Autodesk Fusion 360 part; units mm, degrees
sketch "Sketch1" plane through (0, 0, 0) normal (0, 0, 1) x (1, 0, 0)
  line L0 (40, -70) -> (-40, -70)
  line L1 (-40, -70) -> (-40, 70)
  line L2 (-40, 70) -> (40, 70)
  line L3 (40, 70) -> (40, -70)
  line L4 (40, -70) -> (-40, 70) construction
  line L5 (-40, -70) -> (40, 70) construction
extrude "Extrude1" add sketch "Sketch1" along normal blind 60
sketch "Sketch2" plane through (40, 0, 0) normal (1, 0, 0) x (0, 1, 0)
  line L0 (-70, 0) -> (70, 0)
  line L1 (70, 0) -> (70, 60)
  line L2 (70, 60) -> (-70, 60)
  line L3 (-70, 60) -> (-70, 0)
fillet "Fillet1" radius 10 3 edges at (40, 0, 60) (40, -70, 30) (40, 70, 30)
extrude "Extrude2" add sketch "Sketch2" along normal blind 10
extrude "Extrude3" add 1 faces at (-16.6667, 70, 20) along direction (0, 1, 0) blind 20
sketch "Sketch3" plane through (0, 0, 0) normal (1, 0, 0) x (0, 1, 0)
  line L0 (-1.1501, 56.847) -> (-18.8499, 56.847)
  line L1 (-18.8499, 56.847) -> (-18.8499, 63.153)
  line L2 (-18.8499, 63.153) -> (-1.1501, 63.153)
  line L3 (-1.1501, 63.153) -> (-1.1501, 56.847)
  line L4 (-1.1501, 56.847) -> (-18.8499, 63.153) construction
  line L5 (-18.8499, 56.847) -> (-1.1501, 63.153) construction
  point P0 (-10, 60)
extrude "Extrude4" cut sketch "Sketch3" along normal blind 10
fillet "Fillet2" radius 5 1 edges at (50, 0, 60) 1 faces at (50, -23.3333, 40)
sketch "Sketch4" plane through (0, 0, 0) normal (1, 0, 0) x (0, 1, 0)
  line L0 (7.722, -4.2717) -> (-7.722, -4.2717)
  line L1 (-7.722, -4.2717) -> (-7.722, 4.2717)
  line L2 (-7.722, 4.2717) -> (7.722, 4.2717)
  line L3 (7.722, 4.2717) -> (7.722, -4.2717)
  line L4 (7.722, -4.2717) -> (-7.722, 4.2717) construction
  line L5 (-7.722, -4.2717) -> (7.722, 4.2717) construction
extrude "Extrude5" cut sketch "Sketch4" along normal blind 5
fillet "Fillet3" radius 5 1 edges at (30, 90, 30)
Design review of the part built by this model. Coordinates are the model's own, in mm. A direction names the side the tool comes from. Round coordinates to 2 decimals unless told otherwise and drop trailing zeros. Write each loop counter-clockwise with the first axis right and the second up, starting at its lowest first coordinate (ties: lowest second). Pieces come first, ordered by that corner, then holes.
Item 1: For probe 1 along Y at (x, z) = (3.5, 4); probe 2 along Y at (x, z) = (44, 38); probe 3 along X at (y, z) = (54.5, 55.5), list the stretches that pass through material, from the lowest coordinate up.
Item 2: The part is to be moulded in two halves that separate along X. For faces 1 (the flat face through (42, 1, 60)), 2 (the flat face through (30, 77, 30)), 3 (the cylindrical face through (37.15, -0.98, 56.99)), say which applies: +X half, -X half, draft (parallel to the pull), parting line (faces both ways), or undercut.
Item 3: Clearance check with flat-ended pins moving along their axes: pin 1 Ø5.5 at (x, y) = (2.5, 2.5) entering from -Z; pin 2 Ø3.5 at (y, z) = (-13, 58.5) entering from +X; pin 3 Ø2.5 at (x, z) = (43, 19.5) entering from +Y; pin 4 Ø2 at (y, z) = (-2.5, 2.5) entering from +X. State where each tip first meets the part, or that it passes through.
Item 4: We need section C-C on x = 36. Write out the cut boundary in (y, z).
Item 5: We need section A-A on y = 67. Write out the cut boundary in (x, z).
Item 6: For faces 4 (the flat face through (2, 7.722, 2)), 5 (the flat face through (40, -1, 57)), 6 (the flat face through (42, 70, 30)), 7 (the flat face through (5, -1.15, 58)), 8 (the flat face through (-8, 90, 30)), list the 3-axis set-ups (+Z, -Z, +X, -X, +Y, -Y) from which the entire face can be reached by the end or side of a thin tool; tool diameter is ignored.
Item 7: We need section B-B on z = 20.5. Write out the cut boundary in (x, y), and give its area (3 significant figures).
Returned:
1. probe 1: y = -70 to -7.72, 7.72 to 90
1. probe 2: y = -70 to 70
1. probe 3: x = -40 to 38.35, 40 to 49.97
2. face 1: draft
2. face 2: +X half
2. face 3: undercut
3. pin 1: stops at z = 0
3. pin 2: stops at x = 49.68
3. pin 3: stops at y = 70
3. pin 4: stops at x = 49.77
4. outline: (-68, 0) - (68, 0) - (68, 58) - (-68, 58) - close
5. outline: (-40, 0) - (37.14, 0) - (37.14, 57) arc R10 ccw to (30, 60) - (-40, 60) - close; (40, 0) - (45, 0) arc R5 ccw to (49.58, 3) - (49.58, 57) arc R5 ccw to (45, 60) - (40, 60) - close
6. face 4: -Z
6. face 5: none
6. face 6: +Z, -Z, +X, +Y
6. face 7: +Z
6. face 8: +Z, -Z, +X, -X, +Y
7. outline: (-40, -70) - (30, -70) arc R10 ccw to (40, -60) - (40, -70) - (45, -70) arc R5 ccw to (50, -65) - (50, 65) arc R5 ccw to (45, 70) - (40, 70) - (40, 60) arc R10 ccw to (30, 70) - (30, 85) arc R5 ccw to (25, 90) - (-40, 90) - close
7. area: 13,900 mm2
